Can you work these out from the model? Positions are in its coordinate system, mm. Round coordinates to 2 decimals unless told otherwise and drop trailing zeros. Loops run counter-clockwise (first coordinate to the right, second up) from the corner with the lowest first, then second, coordinate; pieces in that order, holes last.
```python
from build123d import *

# Parameters (mm, degrees)
FILLET1_R    = 5
SCALE1_SCALE = 0.277777778


with BuildPart() as part:
    # Sketch2 → Revolve1 (revolve)
    with BuildSketch(Plane.XY, mode=Mode.PRIVATE) as revolve1_sk:
        with BuildLine():
            Line((40.311288741, 270), (60, 270))
            Line((60, 270), (60, 320))
            Line((60, 320), (-60, 320))
            Line((-60, 320), (-60, 270))
            Line((-60, 270), (-40.311288741, 270))
            ThreePointArc((-40.311288741, 270), (0, 295), (40.311288741, 270))
        make_face()
    revolve(revolve1_sk.sketch.rotate(Axis((-83.864002629, 0, 0), (1, 0, 0)), 90), axis=Axis((-83.864002629, 0, 0), (1, 0, 0)))

    # Fillet1
    fillet1_edges = [part.edges().sort_by_distance(p)[0] for p in [
        (-60, 0, -320),
        (60, 0, -320),
    ]]
    fillet(fillet1_edges, radius=FILLET1_R)


with BuildPart() as part_1:
    # Scale1: scaled about (0, 0, 0)
    add(part.part.scale(SCALE1_SCALE))


solid = part_1.part
```
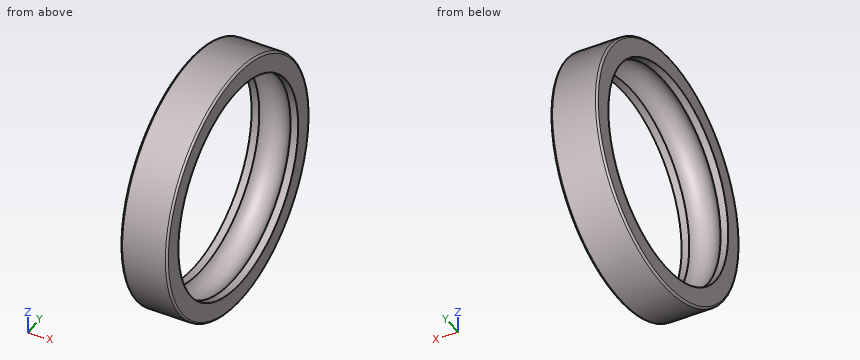
(1) Suppose I cut it at A-A (z = 0). Write out the boundary of the cut face in (x, y).
(2) Suppose I cut it at C-C (x = -0.5). Write out the boundary of the cut face in (y, z), then the cut area to 3 significant figures.
(3) If I drill on line 1 (Y direction, x = 12.9, z = 0); line 2 (Z direction, x = 9.5, y = -36.5); line 3 (Y direction, x = -0.5, z = -62.5), over which ranges is the centre line in solid material (lowest first)?
(4) For pin 1 (1.5 mm diameter, centred on x = 0, y = 10, fed in from +Z); pin 2 (8 mm diameter, centred on x = -13, z = 48.5, fed in from -Y); pin 3 (12 mm diameter, centred on x = -3, y = -65.5, fed in from -Z), each with a flat end and sliding along its axis, tell me the tip position at first contact or that it passes through.
Check result:
1. outline: (-16.67, -87.5) arc R1.39 ccw to (-15.28, -88.89) - (15.28, -88.89) arc R1.39 ccw to (16.67, -87.5) - (16.67, -75) - (11.2, -75) arc R12.5 cw to (-11.2, -75) - (-16.67, -75) - close; (-16.67, 75) - (-11.2, 75) arc R12.5 cw to (11.2, 75) - (16.67, 75) - (16.67, 87.5) arc R1.39 ccw to (15.28, 88.89) - (-15.28, 88.89) arc R1.39 ccw to (-16.67, 87.5) - close
2. outline: circle Ø177.78 at (0, 0); hole circle Ø163.87 at (0, 0)
2. area: 3,730 mm2
3. line 1: y = -88.89 to -75, 75 to 88.89
3. line 2: z = -81.05 to -68.44, 68.44 to 81.05
3. line 3: y = -63.21 to -52.98, 52.98 to 63.21
4. pin 1: stops at z = 88.41
4. pin 2: stops at y = -76.95
4. pin 3: stops at z = -66.04
